```python
from build123d import *

# Parameters (mm, degrees)
SKETCH1_W               = 92
SKETCH1_H               = 92
BOSS_EXTRUDE1_DEPTH     = 2
SKETCH7_R               = 12
BOSS_EXTRUDE2_DEPTH     = 7
BOSS_EXTRUDE2_TAPER     = 15
SKETCH4_R               = 1.7
CUT_EXTRUDE3_DEPTH      = 8.0000001
CUT_EXTRUDE3_DEPTH_BACK = 3
CUT_EXTRUDE4_START      = -0.4
SKETCH6_R               = 3.5
CUT_EXTRUDE4_DEPTH      = 2.6
SKETCH8_W               = 19
SKETCH8_H               = 5
BOSS_EXTRUDE3_DEPTH     = 10
FILLET1_R               = 4
SKETCH12_W              = 7
SKETCH12_H              = 10
BOSS_EXTRUDE6_DEPTH     = 13
SKETCH16_R              = 9.25
CUT_EXTRUDE5_DEPTH      = 60.4
FILLET3_R               = 0.8
SKETCH17_W              = 92
SKETCH17_H              = 92
SKETCH17_W_2            = 88
SKETCH17_H_2            = 88
BOSS_EXTRUDE11_DEPTH    = 30
SKETCH19_R              = 105
SKETCH19_R_2            = 75
CUT_EXTRUDE6_DEPTH      = 92
SKETCH20_W              = 17.4
SKETCH20_H              = 2
BOSS_EXTRUDE12_DEPTH    = 5
SKETCH21_W              = 3
SKETCH21_H              = 20
SKETCH21_W_2            = 1.2
BOSS_EXTRUDE13_DEPTH    = 2
SKETCH22_R              = 1
CUT_EXTRUDE7_DEPTH      = 5
CUT_EXTRUDE8_DEPTH      = 3
BOSS_EXTRUDE14_DEPTH    = 2
SKETCH25_R              = 1
CUT_EXTRUDE9_DEPTH      = 5
SKETCH27_W              = 11
SKETCH27_H              = 5
BOSS_EXTRUDE15_DEPTH    = 6
SKETCH28_R              = 1.15
CUT_EXTRUDE10_DEPTH     = 3
FILLET4_R               = 1
FILLET5_R               = 1
FILLET6_R               = 1


with BuildPart() as part:
    # Sketch1 → Boss-Extrude1 (new body)
    with BuildSketch(Plane(origin=(0, 0, 0), x_dir=(1, 0, 0), z_dir=(0, 1, 0))):
        Rectangle(SKETCH1_W, SKETCH1_H)
    extrude(amount=BOSS_EXTRUDE1_DEPTH)

    # Sketch7 → Boss-Extrude2 (add)
    with BuildSketch(Plane(origin=(0, 2, 0), x_dir=(1, 0, 0), z_dir=(0, 1, 0))):
        Circle(SKETCH7_R)
    extrude(amount=BOSS_EXTRUDE2_DEPTH, taper=BOSS_EXTRUDE2_TAPER)

    # Sketch4 → Cut-Extrude3 (cut, two sides)
    with BuildSketch(Plane(origin=(0, 2, 0), x_dir=(1, 0, 0), z_dir=(0, 1, 0))) as cut_extrude3_sk:
        with Locations((-5.77, 0)):
            Circle(SKETCH4_R)
        with Locations((2.885, 4.99696658)):
            Circle(SKETCH4_R)
        with Locations((2.885, -4.99696658)):
            Circle(SKETCH4_R)
    extrude(amount=CUT_EXTRUDE3_DEPTH, mode=Mode.SUBTRACT)
    extrude(cut_extrude3_sk.sketch, amount=-CUT_EXTRUDE3_DEPTH_BACK, mode=Mode.SUBTRACT)

    # Sketch6 → Cut-Extrude4 (cut, through all)
    with BuildSketch(Plane(origin=(0, 2, 0), x_dir=(1, 0, 0), z_dir=(0, 1, 0)).offset(CUT_EXTRUDE4_START)):
        with Locations((2.885, 4.99696658)):
            Circle(SKETCH6_R)
        with Locations((-5.77, 0)):
            Circle(SKETCH6_R)
        with Locations((2.885, -4.99696658)):
            Circle(SKETCH6_R)
    extrude(amount=-CUT_EXTRUDE4_DEPTH, mode=Mode.SUBTRACT)

    # Sketch8 → Boss-Extrude3 (add)
    with BuildSketch(Plane(origin=(0, 2, 0), x_dir=(1, 0, 0), z_dir=(0, 1, 0))):
        with Locations((-34.5, -35.7)):
            Rectangle(SKETCH8_W, SKETCH8_H)
        with Locations((-34.5, 35.7)):
            Rectangle(SKETCH8_W, SKETCH8_H)
    extrude(amount=BOSS_EXTRUDE3_DEPTH)

    # Fillet1
    fillet1_edges = [part.edges().sort_by_distance(p)[0] for p in [
        (-34.5, 12, -38.2),
        (-34.5, 12, 38.2),
    ]]
    fillet(fillet1_edges, radius=FILLET1_R)

    # Sketch12 → Boss-Extrude6 (add)
    with BuildSketch(Plane(origin=(0, 2, 0), x_dir=(1, 0, 0), z_dir=(0, 1, 0))):
        with Locations((-25.5, 25.2)):
            Rectangle(SKETCH12_W, SKETCH12_H)
        with Locations((-25.5, -25.2)):
            Rectangle(SKETCH12_W, SKETCH12_H)
    extrude(amount=BOSS_EXTRUDE6_DEPTH)

    # Sketch16 → Cut-Extrude5 (cut)
    with BuildSketch(Plane.XY.offset(30.2)):
        with Locations((-34.5, 11.5)):
            Circle(SKETCH16_R)
    extrude(amount=-CUT_EXTRUDE5_DEPTH, mode=Mode.SUBTRACT)

    # Fillet3
    fillet3_edges = [part.edges().sort_by_distance(p)[0] for p in [
        (-22, 15, -25.2),
        (-22, 15, 25.2),
        (-25.937728105, 15, -25.2),
        (-29, 4.06276261, 25.2),
        (-25.937728105, 15, 25.2),
        (-29, 4.06276261, -25.2),
    ]]
    fillet(fillet3_edges, radius=FILLET3_R)

    # Sketch17 → Boss-Extrude11 (add)
    with BuildSketch(Plane(origin=(0, 2, 0), x_dir=(1, 0, 0), z_dir=(0, 1, 0))):
        Rectangle(SKETCH17_W, SKETCH17_H)
        Rectangle(SKETCH17_W_2, SKETCH17_H_2, mode=Mode.SUBTRACT)
    extrude(amount=BOSS_EXTRUDE11_DEPTH)

    # Sketch19 → Cut-Extrude6 (cut)
    with BuildSketch(Plane.XY.offset(46)):
        with Locations((0, -43)):
            Circle(SKETCH19_R)
        with Locations((0, -43)):
            Circle(SKETCH19_R_2, mode=Mode.SUBTRACT)
    extrude(amount=-CUT_EXTRUDE6_DEPTH, mode=Mode.SUBTRACT)

    # Sketch20 → Boss-Extrude12 (add)
    with BuildSketch(Plane(origin=(0, 2, 0), x_dir=(1, 0, 0), z_dir=(0, 1, 0))):
        Polygon((0.6, 44), (0.6, 22), (3.6, 22), (3.6, 42), (20.6, 42), (20.6, 44), align=None)
        with Locations((35.3, 43)):
            Rectangle(SKETCH20_W, SKETCH20_H)
    extrude(amount=BOSS_EXTRUDE12_DEPTH)

    # Sketch21 → Boss-Extrude13 (add)
    with BuildSketch(Plane(origin=(0, 2, 0), x_dir=(1, 0, 0), z_dir=(0, 1, 0))):
        with BuildLine():
            Line((26.6, 44), (20.6, 44))
            Line((20.6, 44), (20.6, 22))
            ThreePointArc((20.6, 22), (23.6, 19), (26.6, 22))
            Line((26.6, 22), (26.6, 44))
        make_face()
        with Locations((42.5, 32)):
            Rectangle(SKETCH21_W, SKETCH21_H)
        with Locations((4.2, 32)):
            Rectangle(SKETCH21_W_2, SKETCH21_H)
    extrude(amount=BOSS_EXTRUDE13_DEPTH)

    # Sketch22 → Cut-Extrude7 (cut, through all)
    with BuildSketch(Plane(origin=(0, 4, 0), x_dir=(1, 0, 0), z_dir=(0, 1, 0))):
        with Locations((23.6, 22)):
            Circle(SKETCH22_R)
        with Locations((23.6, 42)):
            Circle(SKETCH22_R)
    extrude(amount=-CUT_EXTRUDE7_DEPTH, mode=Mode.SUBTRACT)

    # Sketch23 → Cut-Extrude8 (cut, through all)
    with BuildSketch(Plane.ZY.offset(-44)):
        with BuildLine():
            Line((-36, 9.2), (-28, 9.2))
            ThreePointArc((-28, 9.2), (-27.292893219, 8.907106781), (-27, 8.2))
            Line((-27, 8.2), (-27, 5.8))
            ThreePointArc((-27, 5.8), (-27.292893219, 5.092893219), (-28, 4.8))
            Line((-28, 4.8), (-36, 4.8))
            ThreePointArc((-36, 4.8), (-36.707106781, 5.092893219), (-37, 5.8))
            Line((-37, 5.8), (-37, 8.2))
            ThreePointArc((-37, 8.2), (-36.707106781, 8.907106781), (-36, 9.2))
        make_face()
    extrude(amount=-CUT_EXTRUDE8_DEPTH, mode=Mode.SUBTRACT)

    # Sketch24 → Boss-Extrude14 (add)
    with BuildSketch(Plane(origin=(0, 2, 0), x_dir=(1, 0, 0), z_dir=(0, 1, 0))):
        with BuildLine():
            Line((21.6, -44), (25.6, -44))
            Line((25.6, -44), (25.6, -24))
            ThreePointArc((25.6, -24), (23.6, -22), (21.6, -24))
            Line((21.6, -24), (21.6, -44))
        make_face()
        with BuildLine():
            Line((1.6, -44), (5.6, -44))
            Line((5.6, -44), (5.6, -24))
            ThreePointArc((5.6, -24), (3.6, -22), (1.6, -24))
            Line((1.6, -24), (1.6, -44))
        make_face()
        with BuildLine():
            Line((44, 6.5), (37, 6.5))
            ThreePointArc((37, 6.5), (33.5, 3), (37, -0.5))
            Line((37, -0.5), (44, -0.5))
            Line((44, -0.5), (44, 6.5))
        make_face()
    extrude(amount=BOSS_EXTRUDE14_DEPTH)

    # Sketch25 → Cut-Extrude9 (cut, through all)
    with BuildSketch(Plane(origin=(0, 4, 0), x_dir=(1, 0, 0), z_dir=(0, 1, 0))):
        with Locations((3.6, -24)):
            Circle(SKETCH25_R)
        with Locations((23.6, -24)):
            Circle(SKETCH25_R)
        with Locations((37, 3)):
            Circle(SKETCH25_R)
    extrude(amount=-CUT_EXTRUDE9_DEPTH, mode=Mode.SUBTRACT)

    # Sketch27 → Boss-Extrude15 (add)
    with BuildSketch(Plane(origin=(0, 2, 0), x_dir=(1, 0, 0), z_dir=(0, 1, 0))):
        with Locations((-10.9, 41.5)):
            Rectangle(SKETCH27_W, SKETCH27_H)
    extrude(amount=BOSS_EXTRUDE15_DEPTH)

    # Sketch28 → Cut-Extrude10 (cut, through all)
    with BuildSketch(Plane.XY.offset(-44)):
        with Locations((-18.4, 11)):
            Circle(SKETCH28_R)
        with Locations((-3.4, 11)):
            Circle(SKETCH28_R)
        with BuildLine():
            Line((-14.3, 13), (-7.5, 13))
            ThreePointArc((-7.5, 13), (-7.075735931, 12.824264069), (-6.9, 12.4))
            Line((-6.9, 12.4), (-6.9, 9.6))
            ThreePointArc((-6.9, 9.6), (-7.075735931, 9.175735931), (-7.5, 9))
            Line((-7.5, 9), (-14.3, 9))
            ThreePointArc((-14.3, 9), (-14.724264069, 9.175735931), (-14.9, 9.6))
            Line((-14.9, 9.6), (-14.9, 12.4))
            ThreePointArc((-14.9, 12.4), (-14.724264069, 12.824264069), (-14.3, 13))
        make_face()
    extrude(amount=-CUT_EXTRUDE10_DEPTH, mode=Mode.SUBTRACT)

    # Fillet4
    fillet4_edges = [part.edges().sort_by_distance(p)[0] for p in [
        (3.6, 7, -32),
    ]]
    fillet(fillet4_edges, radius=FILLET4_R)

    # Fillet5
    fillet5_edges = [part.edges().sort_by_distance(p)[0] for p in [
        (-16.4, 2, -41.5),
        (-16.4, 5, -44),
        (-10.9, 2, -39),
        (-5.4, 2, -41.5),
        (-5.4, 5, -44),
        (-10.9, 8, -39),
    ]]
    fillet(fillet5_edges, radius=FILLET5_R)

    # Fillet6
    fillet6_edges = [part.edges().sort_by_distance(p)[0] for p in [
        (26.6, 2, -32),
        (23.6, 2, -19),
        (12.7, 2, -42),
        (33.8, 2, -42),
        (42.5, 2, -22),
        (41, 2, -32),
        (20.6, 2, -32),
        (4.8, 2, -32),
        (2.7, 2, -22),
        (0.6, 2, -33),
        (40.5, 2, -6.5),
        (33.5, 2, -3),
        (21.6, 2, 34),
        (23.6, 2, 22),
        (1.6, 2, 34),
        (3.6, 2, 22),
        (40.5, 2, 0.5),
        (25.6, 2, 34),
        (5.6, 2, 34),
        (-34.5, 2, 38.2),
        (-25, 2, 35.7),
        (-25.5, 2, 30.2),
        (-25.5, 2, 20.2),
        (-22, 2, 25.2),
        (-34.5, 2, -38.2),
        (-25, 2, -35.7),
        (-25.5, 2, -30.2),
        (-25.5, 2, -20.2),
        (-22, 2, -25.2),
    ]]
    fillet(fillet6_edges, radius=FILLET6_R)


solid = part.part
```
Input: part model. Units: mm. Frame: model coordinates. A direction names the side the tool comes from. Give positions to 0.01 mm unless a question says otherwise; leave off trailing zeros. Loops run counter-clockwise (first coordinate to the right, second up) from the corner with the lowest first, then second, coordinate; pieces in that order, holes last.
1) Section query B-B on x = -37.5. Return the cut outline in (y, z).
A:
outline: (0, -46) - (21.95, -46) - (21.95, -44) - (2, -44) - (2, -39.2) arc R1 cw to (3, -38.2) - (8, -38.2) arc R4 ccw to (12, -34.2) - (12, -33.2) - (2, -33.2) - (2, 33.2) - (12, 33.2) - (12, 34.2) arc R4 ccw to (8, 38.2) - (3, 38.2) arc R1 cw to (2, 39.2) - (2, 44) - (21.95, 44) - (21.95, 46) - (0, 46) - close
2) Contact query for flat-ended pins moving along their axis: pin 1 (1.6 mm diameter, centred on x = -23.5, z = -26, fed in from +Y); pin 2 (1.5 mm diameter, centred on x = -12, z = -9.5, fed in from +Y); pin 3 (11 mm diameter, centred on x = 2.88, z = 5, fed in from +Y). Output: stop coordinate, or through.
A:
pin 1: stops at y = 15
pin 2: stops at y = 2
pin 3: stops at y = 9
3) Reachability of faces 1 (the flat face through (2, 1.6, 7)), 2 (the cylindrical face through (-25.716, 8.601, -25.13)), 3 (the flat face through (-24, 15, 25)) from +Z, -Z, +X, -X, +Y, -Y: full face, straight path, thin tool, end or side. Return the list, or none.
A:
face 1: -Y
face 2: none
face 3: +Y
4) Line query: L1, parallel to Z at x = -35, y = 4.5; L2, parallel to Z at x = -14.5, y = 23. Output: solid intervals per line, ascending.
A:
L1: z = -46 to -44, -38.2 to -33.2, 33.2 to 38.2, 44 to 46
L2: z = -46 to -44, 44 to 46
5) Section query A-A on y = 25.5. Return the cut outline in (x, z), and give its area (3 significant figures).
A:
outline: (-30.54, -46) - (30.54, -46) - (30.54, -44) - (-30.54, -44) - close; (-30.54, 44) - (30.54, 44) - (30.54, 46) - (-30.54, 46) - close
area: 244 mm2
6) Mould query, pull axis X, two halves, no side actions, for faces 4 (the cylindrical face through (2.516, 5.352, 6.657)), 5 (the flat face through (0, 9, 0)), 6 (the flat face through (-1, 12, -46)). Classes: released by +X, released by -X, zero draft, split by the parting line, or undercut.
A:
face 4: undercut
face 5: undercut
face 6: zero draft
